Source: three-view drawing plus pictorial views. Frame: mm from the lowest corner of the part. Round coordinates to 2 decimals unless told otherwise and drop trailing zeros. Loops run counter-clockwise (first coordinate to the right, second up) from the corner with the lowest first, then second, coordinate; pieces in that order, holes last. Notation, with made-up numbers: M -10,-18 L 27,-18 A20 ccw 27,-5 Z; hole C -30,36 d3. An arc over 180 degrees is marked long. Write each question's results on one line, items separated by ' | '.
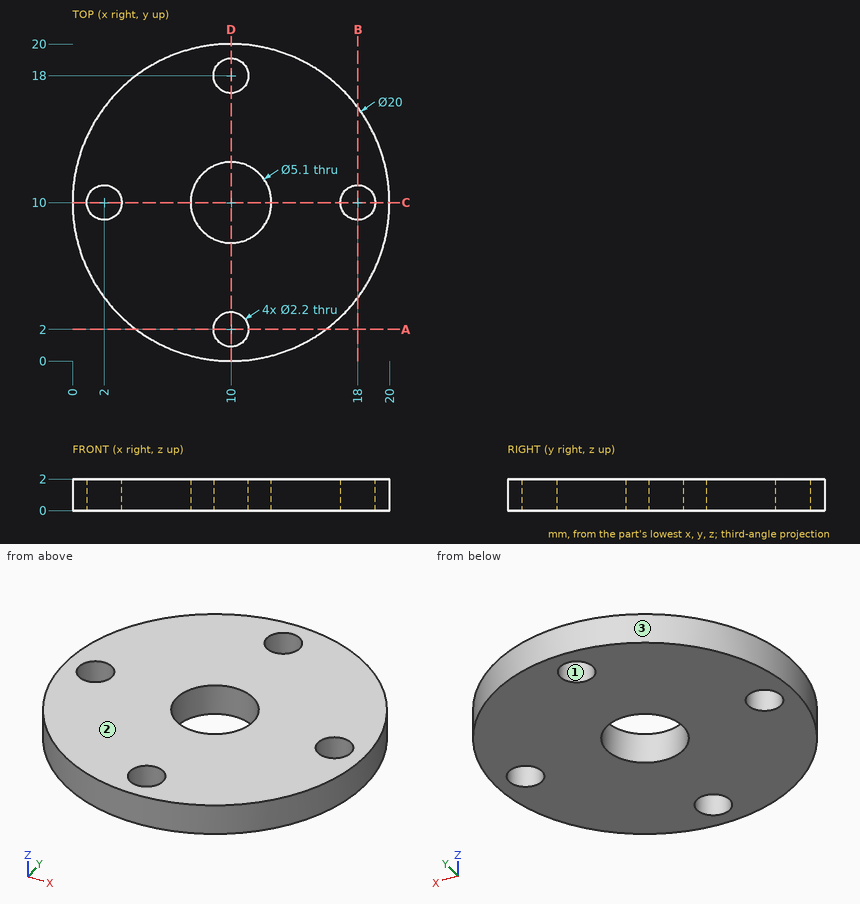
1. Pin query (flat end, axial travel): P1, Ø1.8, axis at x = 10, y = 18, coming from the +Z side. Return the tip coordinate at first contact, or that it passes through.
Answer key:
P1: passes through
2. Ray query, probe 1 along Y at (x, z) = (10, 1.3); probe 2 along Y at (x, z) = (2.25, 1.25); probe 3 along X at (y, z) = (1.5, 1.9). Return the intervals inside material, ascending.
Answer key:
probe 1: y = 0 to 0.9, 3.1 to 7.45, 12.55 to 16.9, 19.1 to 20 | probe 2: y = 3.68 to 8.93, 11.07 to 16.32 | probe 3: x = 4.73 to 9.02, 10.98 to 15.27
3. Draft query along X for the marked faces 1, 2 and 3. Return one class per face: pulls with the +X half, pulls with the -X half, needs draft (parallel to the pull), parting line crosses it, or undercut.
Answer key:
face 1: undercut | face 2: needs draft | face 3: parting line crosses it
4. Section A-A (y = 2). Output: boundary loops of the cut face in (x, z).
Answer key:
outline: M 4,0 L 8.9,0 L 8.9,2 L 4,2 Z; M 11.1,0 L 16,0 L 16,2 L 11.1,2 Z
5. Section C-C (y = 10). Output: boundary loops of the cut face in (x, z).
Answer key:
outline: M 0,0 L 0.9,0 L 0.9,2 L 0,2 Z; M 3.1,0 L 7.45,0 L 7.45,2 L 3.1,2 Z; M 12.55,0 L 16.9,0 L 16.9,2 L 12.55,2 Z; M 19.1,0 L 20,0 L 20,2 L 19.1,2 Z
